Check sheet for the modelled part. Datum: model origin and axes. Units: mm. Face numbers are marked on the shaded views. A direction names the side the tool comes from. Give positions to 0.01 mm unless a question says otherwise; leave off trailing zeros. Write each loop counter-clockwise with the first axis right and the second up, starting at its lowest first coordinate (ties: lowest second). Pieces come first, ordered by that corner, then holes. Notation, with made-up numbers: (20, -8) -> (51, -8) arc R27 ccw to (51, 26) -> close; hole circle Ø4 at (-6.5, 62). An arc over 180 degrees is marked (long way). Return JSON: item names as keys, results as strings.
from build123d import *

# Parameters (mm, degrees)
BOSS_EXTRUDE1_DEPTH         = 15
CUT_EXTRUDE2_DEPTH          = 11
CUT_EXTRUDE2_DEPTH_BACK     = 3
M3_CLEARANCE_HOLE1_D        = 3.4
M3_CLEARANCE_HOLE1_DEPTH    = 3.9
M3_CLEARANCE_HOLE1_TIP      = 1.021463052
TAP_DRILL_FOR_M3X0_5_TAP1_D = 2.5
CHAMFER2_SIZE               = 2.5
FILLET1_R                   = 2


with BuildPart() as part:
    # Sketch1 → Boss-Extrude1 (new body)
    with BuildSketch(Plane(origin=(0, 0, 0), x_dir=(1, 0, 0), z_dir=(0, 1, 0))):
        Polygon((0, 0), (8, 0), (8, 10), (17, 10), (17, 0), (25, 0), (25, -2), (0, -2), align=None)
    extrude(amount=BOSS_EXTRUDE1_DEPTH)

    # Sketch5 → Cut-Extrude2 (cut, two sides)
    with BuildSketch(Plane(origin=(0, 0, 0), x_dir=(-1, 0, 0), z_dir=(0, 0, -1))) as cut_extrude2_sk:
        Polygon((-25, 7.5), (-17, 7.5), (-17, 2), (-8, 2), (-8, 7.5), (0, 7.5), (0, 0), (-8, 0), (-17, 0), (-25, 0), align=None)
    extrude(amount=CUT_EXTRUDE2_DEPTH, mode=Mode.SUBTRACT)
    extrude(cut_extrude2_sk.sketch, amount=-CUT_EXTRUDE2_DEPTH_BACK, mode=Mode.SUBTRACT)

    # M3 Clearance Hole1
    with Locations(Plane(origin=(0, 0, 0), x_dir=(-1, 0, 0), z_dir=(0, 0, -1))):
        with Locations((-4, 11.25), (-21, 11.25)):
            Hole(M3_CLEARANCE_HOLE1_D / 2, depth=M3_CLEARANCE_HOLE1_DEPTH)
            with Locations((0, 0, -(M3_CLEARANCE_HOLE1_DEPTH + M3_CLEARANCE_HOLE1_TIP / 2))):  # 118° drill point
                Cone(0, M3_CLEARANCE_HOLE1_D / 2, M3_CLEARANCE_HOLE1_TIP, mode=Mode.SUBTRACT)

    # Tap Drill for M3x0.5 Tap1 (through all)
    with Locations(Plane.ZY.offset(-8)):
        with Locations((-6, 5.25)):
            Hole(TAP_DRILL_FOR_M3X0_5_TAP1_D / 2)

    # Chamfer2
    chamfer2_edges = [part.edges().sort_by_distance(p)[0] for p in [
        (12.5, 15, -10),
        (12.5, 2, -10),
    ]]
    chamfer(chamfer2_edges, length=CHAMFER2_SIZE)

    # Fillet1
    fillet1_edges = [part.edges().sort_by_distance(p)[0] for p in [
        (17, 7.5, 1),
        (8, 7.5, 1),
    ]]
    fillet(fillet1_edges, radius=FILLET1_R)


solid = part.part
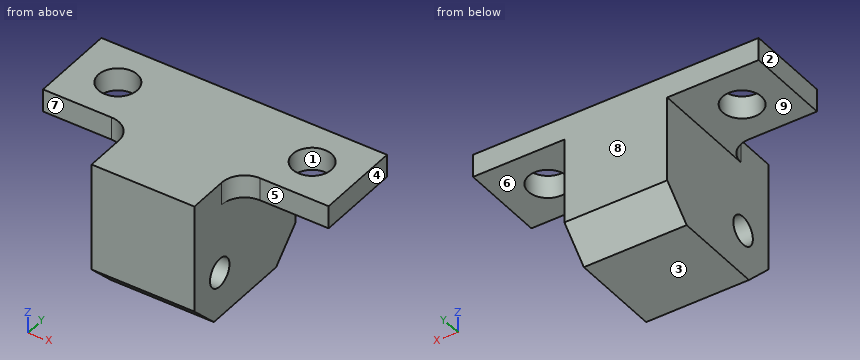
(1) Thickness scan on L1, parallel to Y at x = 12, z = -7; L2, parallel to Y at x = 11, z = -6; L3, parallel to Z at x = 4, y = 13.25. Record the ranges inside material, lowest first.
Reply:
{"L1": "2 to 4.5, 6 to 15", "L2": "2 to 4, 6.5 to 15", "L3": "0 to 2"}
(2) Cross-section at C-C on y = 11.25. Enter the section's corners in (x, z), then the cut area to 3 significant figures.
Reply:
{"outline": "(0, 0) -> (2.3, 0) -> (2.3, 2) -> (0, 2) -> close; (5.7, 0) -> (8, 0) -> (8, -10) -> (17, -10) -> (17, 0) -> (19.3, 0) -> (19.3, 2) -> (5.7, 2) -> close; (22.7, 0) -> (25, 0) -> (25, 2) -> (22.7, 2) -> close", "area": "126 mm^2"}
(3) Cross-section at A-A on x = 9.75. Enter the section's corners in (y, z).
Reply:
{"outline": "(2, -7.5) -> (4.5, -10) -> (12.5, -10) -> (15, -7.5) -> (15, 2) -> (2, 2) -> close; hole circle Ø2.5 at (5.25, -6)"}
(4) Depth check by flat-ended pin: pin 1 Ø5.5 at (x, y) = (21, 11.25) entering from -Z; pin 2 Ø1 at (x, z) = (3, 0.5) entering from -Y; pin 3 Ø3.5 at (y, z) = (7, -3) entering from -X. Enter the tip coordinate at first touch or a pass-through.
Reply:
{"pin 1": "z = 0", "pin 2": "y = 7.5", "pin 3": "x = 8"}
(5) Release check for a two-part mould opening along X. For the marked faces 1, 2, 3 and 4 record: pulls with the +X half, pulls with the -X half, needs draft (parallel to the pull), parting line crosses it, or undercut.
Reply:
{"face 1": "undercut", "face 2": "pulls with the -X half", "face 3": "needs draft", "face 4": "pulls with the +X half"}
(6) Cross-section at B-B on z = -6. Enter the section's corners in (x, y), then the cut area to 3 significant figures.
Reply:
{"outline": "(8, 2) -> (17, 2) -> (17, 4) -> (8, 4) -> close; (8, 6.5) -> (17, 6.5) -> (17, 15) -> (8, 15) -> close", "area": "94.5 mm^2"}
(7) Cross-section at D-D on x = 4. Enter the section's corners in (y, z).
Reply:
{"outline": "(7.5, 0) -> (9.55, 0) -> (9.55, 2) -> (7.5, 2) -> close; (12.95, 0) -> (15, 0) -> (15, 2) -> (12.95, 2) -> close"}
(8) Set-up check for the marked faces 5, 6, 7, 8 and 9: record each of +Z, -Z, +X, -X, +Y, -Y from which the full face is reachable in a straight line by a thin tool's end or side.
Reply:
{"face 5": "+Z, -Z, +X, -Y", "face 6": "-Z, +X, +Y, -Y", "face 7": "+Z, -Z, -X, -Y", "face 8": "+Z, -Z, +X, -X, +Y", "face 9": "-Z, -X, +Y, -Y"}
